```python
from build123d import *

# Parameters (mm, degrees)
F0_W     = 15
F0_H     = 1.4
F0_H_2   = 1.6
F1_DEPTH = 9.75
F2_SIZE  = 0.5
F3_DEPTH = 3.32
F4_DEPTH = 1.25


with BuildPart() as f1:
    # F0 (on Top) → F1 (new body)
    with BuildSketch(Plane.XY):
        with Locations((62.019782, 3.047612)):
            Rectangle(F0_W, F0_H)
        with Locations((62.019782, 6.047612)):
            Rectangle(F0_W, F0_H)
        with Locations((62.019782, 0.047612)):
            Rectangle(F0_W, F0_H)
        with Locations((62.019782, 9.047612)):
            Rectangle(F0_W, F0_H)
        with Locations((62.019782, 4.547612)):
            Rectangle(F0_W, F0_H_2)
        with Locations((62.019782, 1.547612)):
            Rectangle(F0_W, F0_H_2)
        with Locations((62.019782, 7.547612)):
            Rectangle(F0_W, F0_H_2)
        with BuildLine():
            Line((44.519782, 15.147612), (-42.980218, 15.147612))
            Line((-42.980218, 15.147612), (-42.980218, -6.052388))
            Line((-42.980218, -6.052388), (44.519782, -6.052388))
            Line((44.519782, -6.052388), (46.519782, -6.052388))
            Line((46.519782, -6.052388), (46.519782, -5.202388))
            Line((46.519782, -5.202388), (53.519782, -5.202388))
            ThreePointArc((53.519782, -5.202388), (53.812675, -4.495281), (54.519782, -4.202388))
            Line((54.519782, -4.202388), (54.519782, -0.652388))
            Line((54.519782, -0.652388), (54.519782, 0.747612))
            Line((54.519782, 0.747612), (54.519782, 2.347612))
            Line((54.519782, 2.347612), (54.519782, 3.747612))
            Line((54.519782, 3.747612), (54.519782, 5.347612))
            Line((54.519782, 5.347612), (54.519782, 6.747612))
            Line((54.519782, 6.747612), (54.519782, 8.347612))
            Line((54.519782, 8.347612), (54.519782, 9.747612))
            Line((54.519782, 9.747612), (54.519782, 13.297612))
            ThreePointArc((54.519782, 13.297612), (53.812675, 13.590505), (53.519782, 14.297612))
            Line((53.519782, 14.297612), (46.519782, 14.297612))
            Line((46.519782, 14.297612), (46.519782, 15.147612))
            Line((46.519782, 15.147612), (44.519782, 15.147612))
        make_face()
        with BuildLine():
            Line((46.519782, -6.052388), (44.519782, -6.052388))
            ThreePointArc((44.519782, -6.052388), (45.519782, -7.052388), (46.519782, -6.052388))
        make_face()
        with BuildLine():
            ThreePointArc((46.519782, 15.147612), (45.519782, 16.147612), (44.519782, 15.147612))
            Line((44.519782, 15.147612), (46.519782, 15.147612))
        make_face()
        with BuildLine():
            Line((69.519782, 19.047612), (-42.980218, 19.047612))
            Line((-42.980218, 19.047612), (-42.980218, 15.147612))
            Line((-42.980218, 15.147612), (44.519782, 15.147612))
            ThreePointArc((44.519782, 15.147612), (45.519782, 16.147612), (46.519782, 15.147612))
            Line((46.519782, 15.147612), (46.519782, 14.297612))
            Line((46.519782, 14.297612), (53.519782, 14.297612))
            ThreePointArc((53.519782, 14.297612), (54.519782, 15.297612), (55.519782, 14.297612))
            ThreePointArc((55.519782, 14.297612), (55.226889, 13.590505), (54.519782, 13.297612))
            Line((54.519782, 13.297612), (54.519782, 9.747612))
            Line((54.519782, 9.747612), (69.519782, 9.747612))
            Line((69.519782, 9.747612), (69.519782, 19.047612))
        make_face()
        with BuildLine():
            Line((44.519782, -6.052388), (-42.980218, -6.052388))
            Line((-42.980218, -6.052388), (-42.980218, -9.952388))
            Line((-42.980218, -9.952388), (69.519782, -9.952388))
            Line((69.519782, -9.952388), (69.519782, -0.652388))
            Line((69.519782, -0.652388), (54.519782, -0.652388))
            Line((54.519782, -0.652388), (54.519782, -4.202388))
            ThreePointArc((54.519782, -4.202388), (55.226889, -4.495281), (55.519782, -5.202388))
            ThreePointArc((55.519782, -5.202388), (54.519782, -6.202388), (53.519782, -5.202388))
            Line((53.519782, -5.202388), (46.519782, -5.202388))
            Line((46.519782, -5.202388), (46.519782, -6.052388))
            ThreePointArc((46.519782, -6.052388), (45.519782, -7.052388), (44.519782, -6.052388))
        make_face()
        with BuildLine():
            Line((54.519782, -5.202388), (53.519782, -5.202388))
            ThreePointArc((53.519782, -5.202388), (54.519782, -6.202388), (55.519782, -5.202388))
            ThreePointArc((55.519782, -5.202388), (55.226889, -4.495281), (54.519782, -4.202388))
            Line((54.519782, -4.202388), (54.519782, -5.202388))
        make_face()
        with BuildLine():
            ThreePointArc((54.519782, -4.202388), (53.812675, -4.495281), (53.519782, -5.202388))
            Line((53.519782, -5.202388), (54.519782, -5.202388))
            Line((54.519782, -5.202388), (54.519782, -4.202388))
        make_face()
        with BuildLine():
            Line((54.519782, 14.297612), (54.519782, 13.297612))
            ThreePointArc((54.519782, 13.297612), (55.226889, 13.590505), (55.519782, 14.297612))
            ThreePointArc((55.519782, 14.297612), (54.519782, 15.297612), (53.519782, 14.297612))
            Line((53.519782, 14.297612), (54.519782, 14.297612))
        make_face()
        with BuildLine():
            ThreePointArc((53.519782, 14.297612), (53.812675, 13.590505), (54.519782, 13.297612))
            Line((54.519782, 13.297612), (54.519782, 14.297612))
            Line((54.519782, 14.297612), (53.519782, 14.297612))
        make_face()
    extrude(amount=-F1_DEPTH)

    # F2
    f2_edges = [f1.edges().sort_by_distance(p)[0] for p in [
        (13.269782, 19.047612, 0),
        (-42.980218, 4.547612, 0),
        (13.269782, -9.952388, 0),
        (69.519782, 4.547612, 0),
        (-42.980218, 19.047612, -4.875),
        (-42.980218, -9.952388, -4.875),
        (69.519782, 19.047612, -4.875),
        (69.519782, -9.952388, -4.875),
    ]]
    chamfer(f2_edges, length=F2_SIZE)

    # F0 (on Top) → F3 (cut)
    with BuildSketch(Plane.XY):
        with BuildLine():
            Line((44.519782, 15.147612), (-42.980218, 15.147612))
            Line((-42.980218, 15.147612), (-42.980218, -6.052388))
            Line((-42.980218, -6.052388), (44.519782, -6.052388))
            Line((44.519782, -6.052388), (46.519782, -6.052388))
            Line((46.519782, -6.052388), (46.519782, -5.202388))
            Line((46.519782, -5.202388), (53.519782, -5.202388))
            ThreePointArc((53.519782, -5.202388), (53.812675, -4.495281), (54.519782, -4.202388))
            Line((54.519782, -4.202388), (54.519782, -0.652388))
            Line((54.519782, -0.652388), (54.519782, 0.747612))
            Line((54.519782, 0.747612), (54.519782, 2.347612))
            Line((54.519782, 2.347612), (54.519782, 3.747612))
            Line((54.519782, 3.747612), (54.519782, 5.347612))
            Line((54.519782, 5.347612), (54.519782, 6.747612))
            Line((54.519782, 6.747612), (54.519782, 8.347612))
            Line((54.519782, 8.347612), (54.519782, 9.747612))
            Line((54.519782, 9.747612), (54.519782, 13.297612))
            ThreePointArc((54.519782, 13.297612), (53.812675, 13.590505), (53.519782, 14.297612))
            Line((53.519782, 14.297612), (46.519782, 14.297612))
            Line((46.519782, 14.297612), (46.519782, 15.147612))
            Line((46.519782, 15.147612), (44.519782, 15.147612))
        make_face()
        with BuildLine():
            Line((46.519782, -6.052388), (44.519782, -6.052388))
            ThreePointArc((44.519782, -6.052388), (45.519782, -7.052388), (46.519782, -6.052388))
        make_face()
        with BuildLine():
            ThreePointArc((54.519782, -4.202388), (53.812675, -4.495281), (53.519782, -5.202388))
            Line((53.519782, -5.202388), (54.519782, -5.202388))
            Line((54.519782, -5.202388), (54.519782, -4.202388))
        make_face()
        with BuildLine():
            Line((54.519782, -5.202388), (53.519782, -5.202388))
            ThreePointArc((53.519782, -5.202388), (54.519782, -6.202388), (55.519782, -5.202388))
            ThreePointArc((55.519782, -5.202388), (55.226889, -4.495281), (54.519782, -4.202388))
            Line((54.519782, -4.202388), (54.519782, -5.202388))
        make_face()
        with BuildLine():
            ThreePointArc((53.519782, 14.297612), (53.812675, 13.590505), (54.519782, 13.297612))
            Line((54.519782, 13.297612), (54.519782, 14.297612))
            Line((54.519782, 14.297612), (53.519782, 14.297612))
        make_face()
        with BuildLine():
            Line((54.519782, 14.297612), (54.519782, 13.297612))
            ThreePointArc((54.519782, 13.297612), (55.226889, 13.590505), (55.519782, 14.297612))
            ThreePointArc((55.519782, 14.297612), (54.519782, 15.297612), (53.519782, 14.297612))
            Line((53.519782, 14.297612), (54.519782, 14.297612))
        make_face()
        with BuildLine():
            ThreePointArc((46.519782, 15.147612), (45.519782, 16.147612), (44.519782, 15.147612))
            Line((44.519782, 15.147612), (46.519782, 15.147612))
        make_face()
    extrude(amount=-F3_DEPTH, mode=Mode.SUBTRACT)

    # F0 (on Top) → F4 (cut)
    with BuildSketch(Plane.XY):
        with Locations((62.019782, 9.047612)):
            Rectangle(F0_W, F0_H)
        with Locations((62.019782, 6.047612)):
            Rectangle(F0_W, F0_H)
        with Locations((62.019782, 3.047612)):
            Rectangle(F0_W, F0_H)
        with Locations((62.019782, 0.047612)):
            Rectangle(F0_W, F0_H)
    extrude(amount=-F4_DEPTH, mode=Mode.SUBTRACT)


solid = f1.part
```
CAD build for the part. Positions are in the model's coordinates, mm. A direction names the side the tool comes from. Round coordinates to 2 decimals unless told otherwise and drop trailing zeros. Loops run counter-clockwise (first coordinate to the right, second up) from the corner with the lowest first, then second, coordinate; pieces in that order, holes last. Notation, with made-up numbers: M 83,-17.75 L 134,-17.75 A27 ccw 134,6.25 Z; hole C 20,83 d10. An arc over 180 degrees is marked long. Use a Markdown table: item, result. Add a question column.
(1) Cut at B-B (x = -11.5). Give the cut face in (y, z), and give its area (3 significant figures).
(2) Pull direction Y, two halves, no side cores. Call faces 1 (the face through (12, -9.952, -5)), 2 (the face through (12, 16, 0)), 3 (the face through (0, -6.052, -2)): +Y half, -Y half, draft (parallel to the pull), parting line (faces both ways), or undercut.
(3) Cut at A-A (x = 56.5). Give the cut face in (y, z), and give its area (4 significant figures).
(4) Flat gauge pins, fed straight in: pin 1 (11.5 mm diameter, centred on x = 23, y = 4, fed in from +Z); pin 2 (0.7 mm diameter, centred on y = 14.5, z = -1, fed in from -X); pin 3 (1.1 mm diameter, centred on x = 59.5, y = 6, fed in from +Z). Where does each tip first touch, or does it go through?
(5) Which spindle directions (+Z, -Z, +X, -X, +Y, -Y) get a long thin tool onto all of the face, cutting with end or side? Do faces 4 (the face through (50, -5.202, -2)), 5 (the face through (45.542, 16.147, -1.637)), 6 (the face through (14, 19.048, -5)). Say none if no direction does.
(6) Drill centre lines: line 1 (Y direction, x = -6, z = -3); line 2 (Z direction, x = -29, y = -0.25); line 3 (Z direction, x = 57, y = 3). Where is each one in solid material? Low to high.
Geometry says:
| question | item | result |
|---|---|---|
| 1 | outline | M -9.95,-9.75 L 19.05,-9.75 L 19.05,-0.5 L 18.55,0 L 15.15,0 L 15.15,-3.32 L -6.05,-3.32 L -6.05,0 L -9.45,0 L -9.95,-0.5 Z |
| 1 | area | 212 mm² |
| 2 | face 1 | -Y half |
| 2 | face 2 | draft |
| 2 | face 3 | undercut |
| 3 | outline | M -9.95,-9.75 L 19.05,-9.75 L 19.05,-0.5 L 18.55,0 L 9.75,0 L 9.75,-1.25 L 8.35,-1.25 L 8.35,0 L 6.75,0 L 6.75,-1.25 L 5.35,-1.25 L 5.35,0 L 3.75,0 L 3.75,-1.25 L 2.35,-1.25 L 2.35,0 L 0.75,0 L 0.75,-1.25 L -0.65,-1.25 L -0.65,0 L -9.45,0 L -9.95,-0.5 Z |
| 3 | area | 275.5 mm² |
| 4 | pin 1 | stops at z = -3.32 |
| 4 | pin 2 | stops at x = 46.52 |
| 4 | pin 3 | stops at z = -1.25 |
| 5 | face 4 | +Z, -X |
| 5 | face 5 | +Z |
| 5 | face 6 | +Z, -Z, +X, -X, +Y |
| 6 | line 1 | y = -9.95 to -6.05, 15.15 to 19.05 |
| 6 | line 2 | z = -9.75 to -3.32 |
| 6 | line 3 | z = -9.75 to -1.25 |
